The model under review builds one solid part; all positions refer to its coordinate system, in mm. Face numbers are marked on the shaded views. A direction names the side the tool comes from. Round coordinates to 2 decimals unless told otherwise and drop trailing zeros. Write each loop counter-clockwise with the first axis right and the second up, starting at its lowest first coordinate (ties: lowest second). Pieces come first, ordered by that corner, then holes. Notation, with made-up numbers: (19.5, 17.5) -> (59.5, 17.5) arc R32 cw to (59.5, 54.5) -> close; hole circle Ø11 at (-17.5, 6). An arc over 180 degrees is marked (long way). Return JSON: item names as keys, results as strings. Group by question number.
1. Take a section at A-A, the plane y = 0. Write out the cut boundary in (x, z).
2. For line 1 along Z through (x, y) = (-20, -22); line 2 along X through (y, z) = (-1, 13.25); line 3 along Z through (x, y) = (5, -11), list the stretches that pass through material, from the lowest coordinate up. Write a range as from..to.
3. Take a section at C-C, the plane z = 17. Write out the cut boundary in (x, y).
4. Tool access review of the marked faces 1, 2 and 3: name each direction out of +Z, -Z, +X, -X, +Y, -Y from which nothing blocks a thin tool from reaching the whole face with its end or side.
5. Take a section at B-B, the plane y = -21. Write out the cut boundary in (x, z), then the cut area to 3 significant figures.
6. Mouldability with a two-part tool opening along Z and no side actions: class the marked faces 4, 5, 6 and 7 as pulls with the +Z half, pulls with the -Z half, needs draft (parallel to the pull), parting line crosses it, or undercut.
7. Clearance check with flat-ended pins moving along their axes: P1, Ø6, axis at x = 14.5, y = 14, coming from the -Z side; P2, Ø1.5, axis at y = -34, z = 2.5, coming from the +X side; P3, Ø7, axis at x = -21.58, y = 10.51, coming from the -Z side. State where each tip first meets the part, or that it passes through.
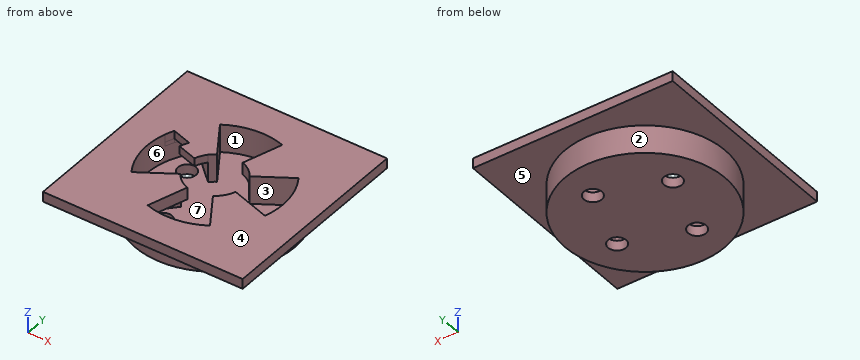
Autodesk Inventor part; units mm, degrees
ref_plane "YZ Plane" through (0, 0, 0) normal (1, 0, 0) x (0, 1, 0)
ref_plane "XZ Plane" through (0, 0, 0) normal (0, 1, 0) x (-1, 0, 0)
ref_plane "XY Plane" through (0, 0, 0) normal (0, 0, 1) x (1, 0, 0)
sketch "Sketch5" plane through (0, 0, 0) normal (0, 0, 1) x (1, 0, 0)
  circle A0 centre (0, 0) radius 34
  dimension "d9" = 68
extrude "Extrusion4" add sketch "Sketch5" along normal blind 5
sketch "Sketch6" plane through (0, 0, 5) normal (0, 0, 1) x (1, 0, 0)
  line L0 (0, 0) -> (-25.0441, 22.9955) construction
  circle A0 centre (0, 0) radius 34 construction
  line L1 (0, 0) -> (-18.239, 28.6939) construction
  line L2 (-25.0441, 22.9955) -> (-10.3123, 9.4687)
  line L3 (-18.239, 28.6939) -> (-7.5102, 11.8151)
  arc A1 (-7.5102, 11.8151) -> (-10.3123, 9.4687) centre (0, 0) ccw
  arc A2 (-18.239, 28.6939) -> (-25.0441, 22.9955) centre (0, 0) ccw
  dimension "d12" = 15
  dimension "d14" = 20
extrude "Extrusion5" add sketch "Sketch6" along normal blind 14
sketch "Sketch7" plane through (-10.3123, 9.4687, 5) normal (-0.6763389, -0.7365906, 0) x (0.7365906, -0.6763389, 0)
  line L0 (-20, 14) -> (0, 14)
  line L1 (0, 14) -> (0, 8)
  line L2 (0, 8) -> (-20, 8)
  line L3 (-20, 8) -> (-20, 14)
  line L4 (14, -8.8) -> (14, 17.8)
  point P0 (14, -5)
  dimension "d17" = 6
  dimension "d18" = 20
revolve "Revolution1" add sketch "Sketch7" angle 25 about axis through (0, 0, 5) along (0, 0, 1)
sketch "Sketch8" plane through (0, 0, 5) normal (0, 0, 1) x (1, 0, 0)
  circle A0 centre (-21.5775, 10.5076) radius 4.5
  circle A1 centre (0, 0) radius 24 construction
  dimension "d25" = 48
  dimension "d21" = 9
extrude "Extrusion6" cut sketch "Sketch8" against normal up to surface (5 mm away)
pattern_circular "Circular Pattern1" count 4 over 360 about axis through (0, 0, 5) along (0, 0, 1) of "Extrusion6", "Revolution1", "Extrusion5"
sketch "Sketch9" plane through (0, 0, 0) normal (0, 0, -1) x (-1, 0, 0)
  circle A0 centre (0, 0) radius 34
  circle A1 centre (0, 0) radius 40
  dimension "d31" = 68
  dimension "d32" = 6
extrude "Extrusion7" add sketch "Sketch9" against normal blind 19
sketch "Sketch10" plane through (0, 0, 19) normal (0, 0, 1) x (1, 0, 0)
  circle A0 centre (0, 0) radius 40
  line L0 (-50, 50) -> (50, 50)
  line L1 (50, 50) -> (50, -50)
  line L2 (50, -50) -> (-50, -50)
  line L3 (-50, -50) -> (-50, 50)
  point P0 (-50, 0)
  point P1 (0, 50)
  dimension "d35" = 100
  dimension "d36" = 100
  dimension "d37" = 80
extrude "Extrusion8" add sketch "Sketch10" against normal blind 5
sketch "Sketch11" plane through (0, 0, 19) normal (0, 0, 1) x (1, 0, 0)
  line L0 (-7.5102, 11.8151) -> (-18.239, 28.6939)
  line L1 (-13.3478, 4.2234) -> (-32.416, 10.2569)
  arc A0 (-12.8746, 20.2545) -> (-22.8819, 7.2402) centre (0, 0) ccw
  arc A1 (-32.416, 10.2569) -> (-28.6939, -18.239) centre (0, 0) ccw
  arc A2 (-18.239, 28.6939) -> (-32.416, 10.2569) centre (0, 0) ccw
  line L2 (-30.7733, 14.4571) -> (-21.1185, 11.4021)
  dimension "d40" = 10
  dimension "d41" = 4.5
extrude "Extrusion9" cut sketch "Sketch11" against normal up to surface (6 mm away) contours A0 L1 A2 L2
sketch "Sketch14" plane through (0, 0, 13) normal (0, 0, -1) x (-0.865517, 0.5008796, 0)
  line L0 (33.1941, 7.3589) -> (13.6681, 3.0302)
  line L1 (13.6681, 3.0302) -> (13.6681, -3.0302)
  line L2 (13.6681, -3.0302) -> (23.4311, -5.1946)
  line L3 (23.4311, -5.1946) -> (13.6681, -3.0302)
  line L4 (23.4311, -5.1946) -> (33.876, -2.9009)
  line L5 (33.876, -2.9009) -> (33.1941, 7.3589)
  point P0 (0, 0)
extrude "Extrusion10" cut sketch "Sketch14" against normal blind 10
sketch "Sketch15" plane through (-10.3123, 9.4687, 5) normal (-0.6763389, -0.7365906, 0) x (0.7365906, -0.6763389, 0)
  line L0 (0, 0) -> (0, 14)
  line L1 (-20, 14) -> (0, 14)
  line L2 (0, 14) -> (0, 10)
  line L3 (0, 10) -> (-20, 10)
  line L4 (-20, 10) -> (-20, 14)
  line L5 (14, -8.8) -> (14, 17.8)
  point P0 (14, -5)
  dimension "d48" = 4
revolve "Revolution2" add sketch "Sketch15" angle 25 about axis through (0, 0, 5) along (0, 0, 1)
sketch "Sketch16" plane through (0, 0, 19) normal (0, 0, 1) x (1, 0, 0)
  line L0 (-32.416, 10.2569) -> (-23.0004, 7.2777)
  line L1 (-13.3478, 4.2234) -> (-32.416, 10.2569)
  line L2 (-21.2392, 11.4403) -> (-30.7733, 14.4571)
  arc A0 (-30.7733, 14.4571) -> (-32.416, 10.2569) centre (0, 0) ccw
  arc A1 (-21.2392, 11.4403) -> (-23.0004, 7.2777) centre (0, 0) ccw
  arc A2 (-32.416, 10.2569) -> (-28.6939, -18.239) centre (0, 0) ccw
  dimension "d50" = 4.5
  dimension "d51" = 10
extrude "Extrusion11" cut sketch "Sketch16" against normal blind 10
properties part number "female 4 bay con"
Output:
{
 "1": {"outline": "(-50, 14) -> (-40, 14) -> (-40, 0) -> (40, 0) -> (40, 14) -> (50, 14) -> (50, 19) -> (34, 19) -> (34, 5) -> (-34, 5) -> (-34, 19) -> (-50, 19) -> close"},
 "2": {"line 1": "z = 0..5, 13..19", "line 2": "x = -39.99..-33.99, 33.99..39.99", "line 3": "z = 0..5"},
 "3": {"outline": "(-50, -50) -> (50, -50) -> (50, 50) -> (-50, 50) -> close; hole (-32.42, 10.26) arc R34 ccw to (-28.69, -18.24) -> (-11.82, -7.51) arc R14 ccw to (-9.47, -10.31) arc R14 ccw to (-4.22, -13.35) -> (-10.26, -32.42) arc R34 ccw to (18.24, -28.69) -> (7.51, -11.82) arc R14 ccw to (10.31, -9.47) arc R14 ccw to (13.35, -4.22) -> (32.42, -10.26) arc R34 ccw to (28.69, 18.24) -> (11.82, 7.51) arc R14 ccw to (9.47, 10.31) arc R14 ccw to (4.22, 13.35) -> (10.26, 32.42) arc R34 ccw to (-18.24, 28.69) -> (-7.51, 11.82) arc R14 ccw to (-10.31, 9.47) arc R14 ccw to (-13.35, 4.22) -> (-23, 7.28) arc R24.12 cw to (-21.24, 11.44) -> (-30.77, 14.46) arc R33.99 ccw to start"},
 "4": {"face 1": "none", "face 2": "-Z", "face 3": "+Z"},
 "5": {"outline": "(-50, 14) -> (-34.04, 14) -> (-34.04, 0) -> (-14.97, 0) -> (-14.97, 5) -> (-19.28, 5) -> (-19.28, 13) -> (-6.64, 13) -> (-6.64, 19) -> (-50, 19) -> close; (-6.04, 0) -> (34.04, 0) -> (34.04, 14) -> (50, 14) -> (50, 19) -> (13.35, 19) -> (13.35, 5) -> (-6.04, 5) -> close; hole (22.87, 5) -> (26.74, 5) -> (26.74, 13) -> (22.87, 13) -> close", "area": "997 mm^2"},
 "6": {"face 4": "pulls with the +Z half", "face 5": "pulls with the -Z half", "face 6": "undercut", "face 7": "undercut"},
 "7": {"P1": "stops at z = 0", "P2": "stops at x = 22.24", "P3": "stops at z = 15"}
}
